Design review of the part built by this model. Coordinates are the model's own, in mm. A direction names the side the tool comes from. Give positions to 0.01 mm unless a question says otherwise; leave off trailing zeros. Order: outer loops, then holes, each group sorted by start corner. A loop starts at its lowest first (then second) coordinate and runs counter-clockwise, first axis right, second up.
```python
from build123d import *

# Parameters (mm, degrees)
SKETCH_R        = 7.5
SKETCH_R_2      = 4
PAD_DEPTH       = 20
SKETCH001_R     = 7.5
SKETCH001_R_2   = 5.7
PAD001_DEPTH    = 20
CHAMFER_SIZE    = 1
CHAMFER001_SIZE = 1
SKETCH002_R     = 5.75
SKETCH002_R_2   = 4.75
PAD002_DEPTH    = 4
CHAMFER002_SIZE = 0.5


with BuildPart() as part:
    # Sketch → Pad (new body)
    with BuildSketch(Plane.XY):
        Circle(SKETCH_R)
        Circle(SKETCH_R_2, mode=Mode.SUBTRACT)
    extrude(amount=PAD_DEPTH)

    # Sketch001 → Pad001 (join)
    with BuildSketch(Plane.XY):
        Circle(SKETCH001_R)
        Circle(SKETCH001_R_2, mode=Mode.SUBTRACT)
    extrude(amount=-PAD001_DEPTH)

    # Chamfer
    chamfer_edges = [part.edges().sort_by_distance(p)[0] for p in [
        (-4, 0, 20),
    ]]
    chamfer(chamfer_edges, length=CHAMFER_SIZE)

    # Chamfer001
    chamfer001_edges = [part.edges().sort_by_distance(p)[0] for p in [
        (-5.7, 0, -20),
    ]]
    chamfer(chamfer001_edges, length=CHAMFER001_SIZE)

    # Sketch002 (on Face6 of Chamfer001) → Pad002 (join)
    with BuildSketch(Plane(origin=(0, 0, 0), x_dir=(1, 0, 0), z_dir=(0, 0, -1))):
        Circle(SKETCH002_R)
        Circle(SKETCH002_R_2, mode=Mode.SUBTRACT)
    extrude(amount=PAD002_DEPTH)

    # Chamfer002
    chamfer002_edges = [part.edges().sort_by_distance(p)[0] for p in [
        (-4.75, 0, -4),
    ]]
    chamfer(chamfer002_edges, length=CHAMFER002_SIZE)


solid = part.part
```
1. Take a section at A-A (y = 0). State the section outline as (x, z) points.
Recorded:
outline: (-7.5, -20) - (-6.7, -20) - (-5.7, -19) - (-5.7, -4) - (-5.25, -4) - (-4.75, -3.5) - (-4.75, 0) - (-4, 0) - (-4, 19) - (-5, 20) - (-7.5, 20) - close; (4, 0) - (4.75, 0) - (4.75, -3.5) - (5.25, -4) - (5.7, -4) - (5.7, -19) - (6.7, -20) - (7.5, -20) - (7.5, 20) - (5, 20) - (4, 19) - close
2. For pin 1 (6 mm diameter, centred on x = -4.5, z = -14.5, fed in from +Y); pin 2 (1.5 mm diameter, centred on y = -3.5, z = -15.5, fed in from +X); pin 3 (3 mm diameter, centred on y = 2, z = 10, fed in from +X); pin 4 (7 mm diameter, centred on x = 0, y = 0, fed in from +Z), all flat-tipped, find the tip position at first contact; note any pin that passes through.
Recorded:
pin 1: stops at y = 7.35
pin 2: stops at x = 6.98
pin 3: stops at x = 7.48
pin 4: passes through
3. Draft analysis for pull direction X (two halves, no side actions). For faces 1 (the face through (2.192, 4.214, -1.726)), 2 (the face through (2, -5, 20)), 3 (the face through (-7.493, 0.33, 0.28)), state which applies: pulls with the +X half, pulls with the -X half, needs draft (parallel to the pull), parting line crosses it, or undercut.
Recorded:
face 1: undercut
face 2: needs draft
face 3: parting line crosses it
4. Take a section at C-C (z = -10). State the section outline as (x, y) points.
Recorded:
outline: circle Ø15 at (0, 0); hole circle Ø11.4 at (0, 0)
5. Machinability: for faces 4 (the face through (-4.5, -3.5, -11.4)), 5 (the face through (0, 7, -20)), which of the approach directions +Z, -Z, +X, -X, +Y, -Y give a long, thin tool a straight path to every point of the face, cutting with its end or side? Answer none if there is none.
Recorded:
face 4: -Z
face 5: -Z, +X, -X, +Y, -Y
6. For line 1 along Y through (x, z) = (0, -8.5); line 2 along Y through (x, z) = (0, 14.75); line 3 along X through (y, z) = (-0.75, 15.5), list the stretches that pass through material, from the lowest coordinate up.
Recorded:
line 1: y = -7.5 to -5.7, 5.7 to 7.5
line 2: y = -7.5 to -4, 4 to 7.5
line 3: x = -7.46 to -3.93, 3.93 to 7.46
